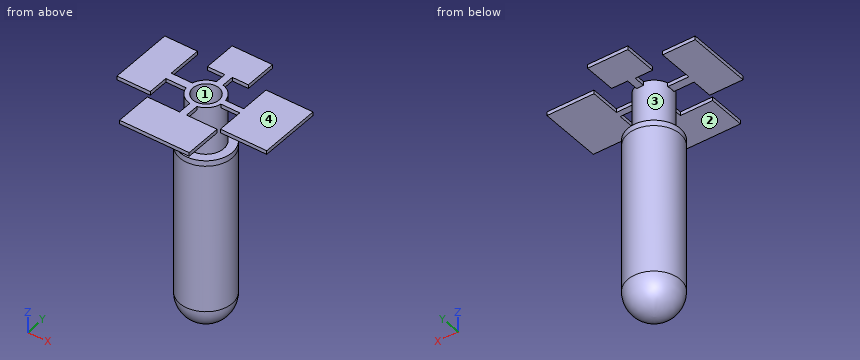
from build123d import *

# Parameters (mm, degrees)
F0_R      = 7
F1_DEPTH  = 7
F2_R      = 6.99999
F5_DEPTH  = 40
F6_R      = 7
F6_R_2    = 5.75
F7_DEPTH  = 1.5
F8_R      = 4.75
F8_R_2    = 3.5
F9_DEPTH  = 12.8
F11_DEPTH = 1


# Not quite as in the source:
# - a fillet or chamfer is up to 0.001 mm smaller than in the source, because OpenCascade refuses the exact size


with BuildPart() as f1:
    # F0 (on Top) → F1 (new body)
    with BuildSketch(Plane.XY):
        Circle(F0_R)
    extrude(amount=-F1_DEPTH)

    # F2 (radius 7 in the source; OpenCascade refuses exactly that, so slightly less here)
    f2_edges = [f1.edges().sort_by_distance(p)[0] for p in [
        (-7, 0, -7),
    ]]
    fillet(f2_edges, radius=F2_R)

    # F3 (on face) → F4 (revolve, cut)
    with BuildSketch(Plane.XY):
        with BuildLine():
            Line((-5.75, 0), (5.75, 0))
            ThreePointArc((5.75, 0), (0, 5.75), (-5.75, 0))
        make_face()
    revolve(axis=Axis((0, 0, 0), (1, 0, 0)), mode=Mode.SUBTRACT)

    # F5 (add): a face of the model
    f5_faces = [f1.faces().sort_by_distance(p)[0] for p in [
        (-6.8020101013, 0, 0),
    ]]
    extrude(f5_faces, amount=F5_DEPTH)

    # F6 (on face) → F7 (join)
    with BuildSketch(Plane.XY.offset(40)):
        Circle(F6_R)
        Circle(F6_R_2, mode=Mode.SUBTRACT)
        Circle(F6_R_2)
    extrude(amount=F7_DEPTH)

    # F8 (on face) → F9 (join)
    with BuildSketch(Plane.XY.offset(41.5)):
        Circle(F8_R)
        Circle(F8_R_2, mode=Mode.SUBTRACT)
    extrude(amount=F9_DEPTH)

    # F10 (on face) → F11 (join)
    with BuildSketch(Plane.XY.offset(54.3)):
        with BuildLine():
            ThreePointArc((-4.6668358831, -0.8849535807), (-4.7461193146, 0.1919673186), (-4.5801202528, 1.2589672237))
            Line((-4.5801202528, 1.2589672237), (-10.254695956, 1.2589672237))
            Line((-10.254695956, 1.2589672237), (-10.254695956, 10.6798189955))
            Line((-10.254695956, 10.6798189955), (-18.9986647217, 10.6798189955))
            Line((-18.9986647217, 10.6798189955), (-18.9986647217, -6.4948128273))
            Line((-18.9986647217, -6.4948128273), (-10.0838066189, -6.4948128273))
            Line((-10.0838066189, -6.4948128273), (-10.0838066189, -0.8849535807))
            Line((-10.0838066189, -0.8849535807), (-4.6668358831, -0.8849535807))
        make_face()
        with BuildLine():
            Line((-0.7236261107, 7.7295311092), (-0.7236261107, 4.6945569814))
            ThreePointArc((-0.7236261107, 4.6945569814), (0.2079220104, 4.7454471273), (1.1314493255, 4.6132767556))
            Line((1.1314493255, 4.6132767556), (1.1314493255, 7.9441230255))
            Line((1.1314493255, 7.9441230255), (5.4202612606, 7.9441230255))
            Line((5.4202612606, 7.9441230255), (5.4202612606, 16.6028177181))
            Line((5.4202612606, 16.6028177181), (-5.3641636993, 16.6028177181))
            Line((-5.3641636993, 16.6028177181), (-5.3641636993, 7.7295311092))
            Line((-5.3641636993, 7.7295311092), (-0.7236261107, 7.7295311092))
        make_face()
        with BuildLine():
            Line((9.5364480238, 0.7383154319), (4.6922692083, 0.7383154319))
            ThreePointArc((4.6922692083, 0.7383154319), (4.7355453086, 0.3702845262), (4.75, 0))
            ThreePointArc((4.75, 0), (4.7285644054, -0.4507534407), (4.6644510887, -0.8974386001))
            Line((4.6644510887, -0.8974386001), (9.7088032833, -0.8974386001))
            Line((9.7088032833, -0.8974386001), (9.7088032833, -7.8623809823))
            Line((9.7088032833, -7.8623809823), (22.1269458032, -7.8623809823))
            Line((22.1269458032, -7.8623809823), (22.1269458032, -5.6407864176))
            Line((22.1269458032, -5.6407864176), (22.1269458032, 8.7704470205))
            Line((22.1269458032, 8.7704470205), (9.5364480238, 8.7704470205))
            Line((9.5364480238, 8.7704470205), (9.5364480238, 0.7383154319))
        make_face()
        with BuildLine():
            ThreePointArc((1.0145288717, -4.6403912732), (0.0864892709, -4.7492125248), (-0.8448971996, -4.6742538145))
            Line((-0.8448971996, -4.6742538145), (-0.8448971996, -8.3471687661))
            Line((-0.8448971996, -8.3471687661), (-9.48290206, -8.3471687661))
            Line((-9.48290206, -8.3471687661), (-9.48290206, -18.3443419333))
            Line((-9.48290206, -18.3443419333), (9.1727929611, -18.3443419333))
            Line((9.1727929611, -18.3443419333), (9.1727929611, -8.3204683216))
            Line((9.1727929611, -8.3204683216), (1.0145288717, -8.3204683216))
            Line((1.0145288717, -8.3204683216), (1.0145288717, -4.6403912732))
        make_face()
    extrude(amount=-F11_DEPTH)


solid = f1.part
Model file for the job. Use its own axes, mm. Face numbers are marked on the shaded views. A direction names the side the tool comes from. Give positions to 0.01 mm unless a question says otherwise; leave off trailing zeros. Order: outer loops, then holes, each group sorted by start corner. A loop starts at its lowest first (then second) coordinate and runs counter-clockwise, first axis right, second up. Notation, with made-up numbers: (85, 21.25) - (118, 21.25) arc R4 ccw to (118, 26.25) - close; hole circle Ø6 at (68.5, -1.75). An arc over 180 degrees is marked (long way). One line per item, written item: value.
Item 1: Slice it at A-A (x = -8). List the corners of the cut face in (y, z).
Response values:
outline: (-18.34, 53.3) - (-8.35, 53.3) - (-8.35, 54.3) - (-18.34, 54.3) - close; (-0.88, 53.3) - (1.26, 53.3) - (1.26, 54.3) - (-0.88, 54.3) - close
Item 2: Wall check: line 1 (Y direction, x = 0, z = 45); line 2 (Y direction, x = 0, z = 15). Give the ranges that are in metal, low to high.
Response values:
line 1: -4.75 to -3.5, 3.5 to 4.75
line 2: -7 to -5.75, 5.75 to 7
Item 3: Pin check, flat tips, straight feed: pin 1 Ø11 at (x, y) = (1.5, -13) entering from -Z; pin 2 Ø0.8 at (x, z) = (6.5, 54) entering from +Y; pin 3 Ø0.5 at (y, z) = (13, 54) entering from +X. Stop position of each tip, or through.
Response values:
pin 1: z = 53.3
pin 2: y = 0.74
pin 3: x = 5.42
Item 4: Slice it at D-D (x = -14). List the corners of the cut face in (y, z), then the cut area to 3 significant figures.
Response values:
outline: (-6.49, 53.3) - (10.68, 53.3) - (10.68, 54.3) - (-6.49, 54.3) - close
area: 17.2 mm2
Item 5: Slice it at B-B (y = -12). List the corners of the cut face in (x, z), then the cut area to 3 significant figures.
Response values:
outline: (-9.48, 53.3) - (9.17, 53.3) - (9.17, 54.3) - (-9.48, 54.3) - close
area: 18.7 mm2
Item 6: Tool access for the marked faces 3 and 4: list every direction of +Z, -Z, +X, -X, +Y, -Y with a clear straight run to the whole face (end or side of a thin tool).
Response values:
face 3: none
face 4: +Z, +X, -X, +Y, -Y
Item 7: Slice it at C-C (z = 4). List the corners of the cut face in (x, y), then the cut area to 3 significant figures.
Response values:
outline: circle Ø14 at (0, 0); hole circle Ø11.5 at (0, 0)
area: 50.1 mm2
Item 8: Two-plate mould, pull along Y, no slides. Class the marked faces 1 and 2: released by +Y, released by -Y, zero draft, split by the parting line, or undercut.
Response values:
face 1: undercut
face 2: zero draft
